Read the model definition and answer for the solid it produces. Units are mm, in the model's axes. A direction names the side the tool comes from. Coordinates: 2 decimals unless noted, no trailing zeros. Order: outer loops, then holes, each group sorted by start corner. A loop starts at its lowest first (then second) coordinate and runs counter-clockwise, first axis right, second up. Notation, with made-up numbers: (8, 24.25) -> (37, 24.25) arc R28 ccw to (37, 61.25) -> close; hole circle Ø9 at (67, 39). An arc over 180 degrees is marked (long way). Use CSV: the item, a comma, the result in double quotes.
```python
from build123d import *

# Parameters (mm, degrees)
SKETCH1_R                         = 30.48
BOSS_EXTRUDE1_DEPTH               = 25.4
SKETCH7_R                         = 11.43
CUT_EXTRUDE2_DEPTH                = 12.7
F_1_4_CLEARANCE_HOLE1_D           = 6.5278
F_1_4_28_TAPPED_HOLE1_D           = 5.4102
F_1_4_NPT_TAPPED_HOLE1_AT_2_COUNT = 2
F_1_4_NPT_TAPPED_HOLE1_AT_2_PITCH = 22.225
SKETCH13_R                        = 17.145
CUT_EXTRUDE3_DEPTH                = 12.7
MOVE_FACE1_BY                     = 12.7
CUT_EXTRUDE4_DEPTH                = 51.032197633
CUT_EXTRUDE4_DEPTH_BACK           = 51.032197633
SKETCH17_R                        = 6.35


with BuildPart() as part:
    # Sketch1 → Boss-Extrude1 (new body)
    with BuildSketch(Plane(origin=(0, 0, 0), x_dir=(1, 0, 0), z_dir=(0, 1, 0))):
        with Locations(Location((0, 0, 0), (0, 0, 270))):
            Circle(SKETCH1_R)
    extrude(amount=BOSS_EXTRUDE1_DEPTH)

    # Sketch7 → Cut-Extrude2 (cut)
    with BuildSketch(Plane.XZ):
        with Locations(Location((0, 0, 0), (0, 0, 270))):
            Circle(SKETCH7_R)
    extrude(amount=-CUT_EXTRUDE2_DEPTH, mode=Mode.SUBTRACT)

    # 1/4 Clearance Hole1 (through all)
    with Locations(Plane(origin=(0, 25.4, 0), x_dir=(1, 0, 0), z_dir=(0, 1, 0))):
        with Locations((20.175514493, 15.615257641), (3.435452557, -25.280136906), (-3.435452557, 25.280136906), (-20.175514493, -15.615257641)):
            Hole(F_1_4_CLEARANCE_HOLE1_D / 2)

    # 1/4-28 Tapped Hole1 (through all)
    with Locations(Plane(origin=(0, 25.4, 0), x_dir=(1, 0, 0), z_dir=(0, 1, 0))):
        with Locations((0, 0)):
            Hole(F_1_4_28_TAPPED_HOLE1_D / 2)

    # Sketch12 → 1/4 NPT Tapped Hole1 (revolve, cut)
    with BuildSketch(Plane(origin=(-10.284247774, 25.4, -4.20973918), x_dir=(0, 0, 1), z_dir=(1, 0, 0))):
        Polygon((0, 0), (0, 25.4), (5.5626, 25.4), (5.5626, 9.906), (6.557984794, 9.906), (6.8545837, 0), align=None)
    f_1_4_npt_tapped_hole1 = revolve(axis=Axis((-10.284247774, 31.75, -4.20973918), (0, -1, 0)), mode=Mode.SUBTRACT)

    # 1/4 NPT Tapped Hole1 at 2: 1/4 NPT Tapped Hole1 ×2
    with Locations(*[Vector(0.9254666163685323, 0, 0.3788291725664483) * (i * F_1_4_NPT_TAPPED_HOLE1_AT_2_PITCH) for i in range(1, F_1_4_NPT_TAPPED_HOLE1_AT_2_COUNT)]):
        add(f_1_4_npt_tapped_hole1, mode=Mode.SUBTRACT)

    # Sketch13 → Cut-Extrude3 (cut)
    with BuildSketch(Plane.XZ):
        with Locations(Location((0, 0, 0), (0, 0, 270))):
            Circle(SKETCH13_R)
    extrude(amount=-CUT_EXTRUDE3_DEPTH, mode=Mode.SUBTRACT)

    # Move Face1: a face moved outward by 12.7
    extrude(part.faces().sort_by_distance((0, 0, 24.384))[0], amount=MOVE_FACE1_BY, dir=(0, -1, 0))

    # Sketch17 → Cut-Extrude4 (cut, two sides: drawn at the far end of the back side and taken through both)
    with BuildSketch(Plane(origin=(0, 0, 0), x_dir=(-0.37882917256642434, 0, 0.9254666163685421), z_dir=(-0.9254666163685421, 0, -0.37882917256642434)).offset(-CUT_EXTRUDE4_DEPTH_BACK)):
        Circle(SKETCH17_R)
    extrude(amount=CUT_EXTRUDE4_DEPTH + CUT_EXTRUDE4_DEPTH_BACK, mode=Mode.SUBTRACT)


solid = part.part
```
Item 1: Find section B-B, the plane z = -23.5. Give the vertices of the cut face in (x, y).
Return value:
outline,"(-19.41, -12.7) -> (-6.17, -12.7) -> (-6.17, 25.4) -> (-19.41, 25.4) -> close; (-0.7, -12.7) -> (19.41, -12.7) -> (19.41, 25.4) -> (-0.7, 25.4) -> close"
Item 2: Each of these flat-tipped pins is pushed along its axis until it touches: P1, Ø4, axis at x = -9, y = 19, coming from the +Z side; P2, Ø6, axis at x = 0, z = 0, coming from the -Y side; P3, Ø4, axis at y = 16, z = -1, coming from the +X side. Where does it stop, or does it pass through?
Return value:
P1,"stops at z = 29.67"
P2,"stops at y = 12.7"
P3,"stops at x = 30.48"
Item 3: The mould has two halves that part along Y. Classify faces 1 (the conical face through (5.75, 20.516, -0.735)), 2 (the flat face through (0, 12.7, -4)), 3 (the cylindrical face through (-2.58, 18.96, -0.81)), 4 (the cylindrical face through (-18.982, 0.279, -14.625)): +Y half, -Y half, draft (parallel to the pull), parting line (faces both ways), or undercut.
Return value:
face 1,"+Y half"
face 2,"-Y half"
face 3,"draft"
face 4,"undercut"
Item 4: Straight lines are drawn through the part: line 1 along Z through (x, y) = (5, 8); line 2 along Z through (x, y) = (2, 23.5); line 3 along X through (y, z) = (19, 1). For each, find the intervals that lie inside material, in ascending order.
Return value:
line 1,"z = -30.07 to -16.4, 16.4 to 22.42, 28.14 to 30.07"
line 2,"z = -30.41 to -1.82, 1.82 to 22.35, 28.21 to 30.41"
line 3,"x = -30.46 to -14.44, -6.13 to -2.51, 2.51 to 4.45, 16.12 to 30.46"
Item 5: Find section A-A, the plane y = -5.5. Give the vertices of the cut face in (x, z) (3 decimals).
Return value:
outline,"(-29.257, -8.547) -> (-16.795, -3.446) arc R17.145 cw to (14.391, 9.32) -> (26.853, 14.421) arc R30.48 ccw to start; (-26.853, -14.421) arc R30.48 ccw to (29.257, 8.547) -> (16.795, 3.446) arc R17.145 cw to (-14.391, -9.32) -> close; hole circle Ø6.528 at (-20.176, 15.615); hole circle Ø6.528 at (-3.435, -25.28); hole circle Ø6.528 at (3.435, 25.28); hole circle Ø6.528 at (20.176, -15.615)"
Item 6: Find section C-C, the plane y = 19.5. Give the vertices of the cut face in (x, z), then the cut area to 3 significant figures.
Return value:
outline,"circle Ø60.96 at (0, 0); hole circle Ø6.53 at (-20.18, 15.62); hole circle Ø13.36 at (-10.28, -4.21); hole circle Ø6.53 at (-3.44, -25.28); hole circle Ø5.41 at (0, 0); hole circle Ø6.53 at (3.44, 25.28); hole circle Ø13.36 at (10.28, 4.21); hole circle Ø6.53 at (20.18, -15.62)"
area,"2,480 mm^2"
Item 7: Find section D-D, the plane x = -19. Give the number of separate pieces and of enclosed holes in the cut face, then the cut area to 3 significant figures.
Return value:
separate pieces,"2"
enclosed holes,"1"
area,"1,450 mm^2"
Item 8: A tool of negligible diameter and unlimited length cuts with its end or side. For faces 5 (the cylindrical face through (20.6, 6.617, -22.465)), 6 (the flat face through (16, 15.494, 6)), from which of +Z, -Z, +X, -X, +Y, -Y can it reach the whole face along a straight path? Write none if from no direction.
Return value:
face 5,"+Y, -Y"
face 6,"+Y"
